Print and shaded views of the part. All mm, measured from the part's lowest x, y and z. Coordinates: 2 decimals unless noted, no trailing zeros. Loops run counter-clockwise (first coordinate to the right, second up) from the corner with the lowest first, then second, coordinate; pieces in that order, holes last. Notation, with made-up numbers: (38.5, 15.5) -> (95.5, 15.5) arc R29 ccw to (95.5, 50.5) -> close; hole circle Ø8 at (80, 28). An arc over 180 degrees is marked (long way). One line per question, with ' | ' between items. Start each with the question number.
1) Cut at C-C (y = 0.8). List the corners of the cut face in (x, z), plus the area to 3 significant figures.
2) Cut at B-B (z = 23). List the corners of the cut face in (x, y).
3) Cut at A-A (x = 25.5). List the corners of the cut face in (y, z), plus the area to 3 significant figures.
4) Drop flat-ended pins along their axis: pin 1 (0.9 mm diameter, centred on x = 104.5, y = 2, fed in from -Z); pin 2 (1 mm diameter, centred on x = 57.5, z = 99, fed in from -Y). Give the stop position or say it passes through.
5) Probe L1, parallel to Z at x = 106, y = 1.8; L2, parallel to X at y = 2.75, z = 91. List the from-to ranges inside material, lowest first. Write a range as from..to.
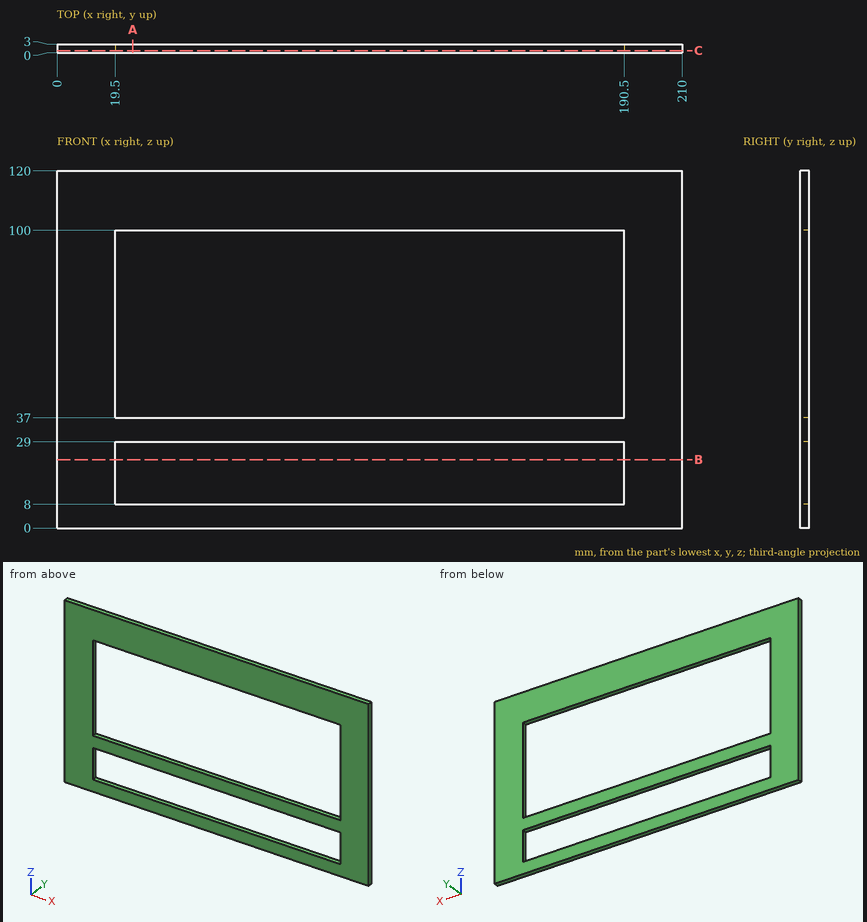
Reported:
1) outline: (0, 0) -> (210, 0) -> (210, 120) -> (0, 120) -> close; hole (19.5, 8) -> (190.5, 8) -> (190.5, 29) -> (19.5, 29) -> close; hole (19.5, 37) -> (190.5, 37) -> (190.5, 100) -> (19.5, 100) -> close | area: 10,800 mm²
2) outline: (0, 0) -> (19.5, 0) -> (19.5, 3) -> (0, 3) -> close; (190.5, 0) -> (210, 0) -> (210, 3) -> (190.5, 3) -> close
3) outline: (0, 0) -> (3, 0) -> (3, 8) -> (0, 8) -> close; (0, 29) -> (3, 29) -> (3, 37) -> (0, 37) -> close; (0, 100) -> (3, 100) -> (3, 120) -> (0, 120) -> close | area: 108 mm²
4) pin 1: stops at z = 0 | pin 2: passes through
5) L1: z = 0..8, 29..37, 100..120 | L2: x = 0..19.5, 190.5..210
